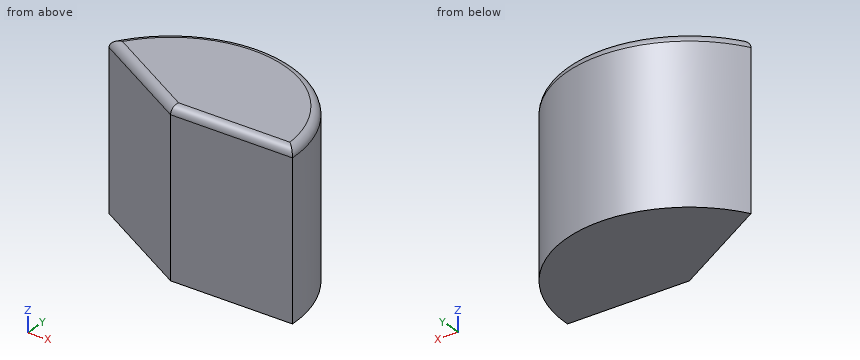
```python
from build123d import *

# Parameters (mm, degrees)
BOSS_EXTRUDE1_DEPTH = 40
FILLET1_R           = 2


with BuildPart() as part:
    # Sketch1 → Boss-Extrude1 (new body)
    with BuildSketch(Plane.XY):
        with BuildLine():
            Line((-25.980762114, 15), (0, 0))
            Line((0, 0), (30, 0))
            ThreePointArc((30, 0), (7.764571353, 28.977774789), (-25.980762114, 15))
        make_face()
    extrude(amount=BOSS_EXTRUDE1_DEPTH)

    # Fillet1
    fillet1_edges = [part.edges().sort_by_distance(p)[0] for p in [
        (-12.990381057, 7.5, 40),
        (15, 0, 40),
        (7.764571353, 28.977774789, 40),
    ]]
    fillet(fillet1_edges, radius=FILLET1_R)


solid = part.part
```
Geometry: final body of the model. Coordinates: model frame, mm. Round coordinates to 2 decimals unless told otherwise and drop trailing zeros. Order: outer loops, then holes, each group sorted by start corner. A loop starts at its lowest first (then second) coordinate and runs counter-clockwise, first axis right, second up. Notation, with made-up numbers: M 16.25,80.5 L 34.25,80.5 A20 cw 34.25,100.5 Z; hole C 24.5,-21 d10. An arc over 180 degrees is marked long. Use one line per item in the form item = value. Start each with the question number.
Q1. Pin query (flat end, axial travel): pin 1 Ø5 at (x, z) = (8.5, 19.5) entering from +Y; pin 2 Ø2 at (y, z) = (12.5, 28) entering from +X; pin 3 Ø2 at (y, z) = (23.5, 24) entering from -X. Return the tip coordinate at first contact, or that it passes through.
Q2. Cut plane A-A (z = 17). Return loops of the section in (x, y), and give its area (3 significant figures).
Q3. Material intervals for line 1 (Y direction, x = -7, z = 29); line 2 (X direction, y = 19, z = 28); line 3 (Y direction, x = 14.5, z = 3), sorted ascending. Write a range as [from, to].
Geometry results:
q1.pin_1 = 29.39
q1.pin_2 = 27.71
q1.pin_3 = -19.84
q2.outline = M -25.98,15 L 0,0 L 30,0 A30 ccw Z
q2.area = 1,180 mm^2
q3.line_1 = [4.04, 29.17]
q3.line_2 = [-23.22, 23.22]
q3.line_3 = [0, 26.26]
